Work out the finished part from the listing and answer in its coordinate system (mm). Face numbers are marked on the shaded views. A direction names the side the tool comes from. Coordinates: 2 decimals unless noted, no trailing zeros. Write each loop counter-clockwise with the first axis right and the second up, starting at its lowest first coordinate (ties: lowest second). Pieces come first, ordered by that corner, then holes. Notation, with made-up numbers: M 62.25,38 L 66.25,38 A17 ccw 66.25,51 Z; hole C 0.5,1 d8. An arc over 180 degrees is marked long. Use CSV: the item, a comma, the result in double quotes.
from build123d import *

# Parameters (mm, degrees)
F0_R     = 12.5
F1_DEPTH = 25
F2_R     = 5


with BuildPart() as f1:
    # F0 (on Front) → F1 (new body)
    with BuildSketch(Plane.XZ):
        with BuildLine():
            ThreePointArc((25.1206115917, 18.3788214192), (0, 57.0683197663), (-25.1206115917, 18.3788214192))
            Line((-25.1206115917, 18.3788214192), (-25.1206115917, -41.6211785808))
            Line((-25.1206115917, -41.6211785808), (25.1206115917, -41.6211785808))
            Line((25.1206115917, -41.6211785808), (25.1206115917, 18.3788214192))
        make_face()
        with Locations((0, 29.5683197663)):
            Circle(F0_R, mode=Mode.SUBTRACT)
    extrude(amount=F1_DEPTH)

    # F2
    f2_edges = [f1.edges().sort_by_distance(p)[0] for p in [
        (-25.120612, -12.5, -41.621179),
        (25.120612, -12.5, -41.621179),
        (-25.120612, -12.5, 18.378821),
        (25.120612, -12.5, 18.378821),
        (0, 0, 57.06832),
        (0, -25, 57.06832),
        (25.120612, 0, -11.621179),
        (25.120612, -25, -11.621179),
        (-25.120612, 0, -11.621179),
        (-25.120612, -25, -11.621179),
    ]]
    fillet(f2_edges, radius=F2_R)


solid = f1.part
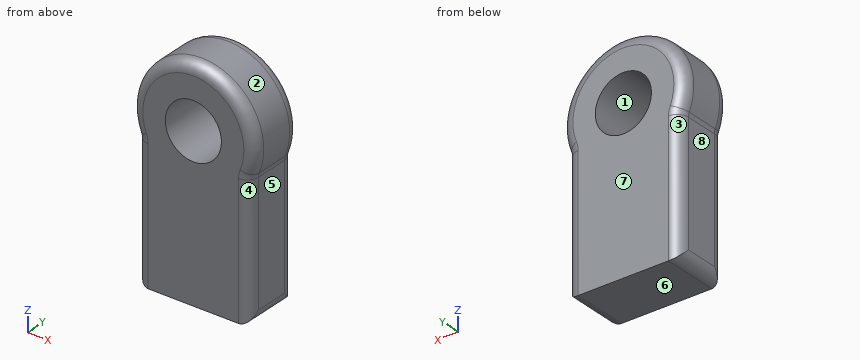
Item 1: Consider probe 1 along Z at (x, y) = (0, -8); probe 2 along X at (y, z) = (-8.25, 2.5); probe 3 along Z at (x, y) = (-10, -4.75). Determine where each line is inside the solid, lowest interval first.
Answer:
probe 1,"z = -41.62 to 17.07, 42.07 to 57.07"
probe 2,"x = -25.12 to 25.12"
probe 3,"z = -41.62 to 22.07, 37.07 to 55.18"
Item 2: A tool of negligible diameter and unlimited length cuts with its end or side. For the marked faces 4, 5, 6, 7 and 8, from which of +Z, -Z, +X, -X, +Y, -Y can it reach the whole face along a straight path? Write none if from no direction.
Answer:
face 4,"-Z, +X, -Y"
face 5,"-Z, +X, +Y, -Y"
face 6,"-Z, +X, -X, +Y, -Y"
face 7,"+Z, -Z, +X, -X, +Y"
face 8,"-Z, -X, +Y, -Y"
Item 3: The part is cut by section A-A (x = 0). Write down the section's boundary in (y, z).
Answer:
outline,"M -25,-41.62 L 0,-41.62 L 0,17.07 L -25,17.07 Z; M -25,42.07 L 0,42.07 L 0,52.07 A5 ccw -5,57.07 L -20,57.07 A5 ccw -25,52.07 Z"
Item 4: For a pull along X with two mould halves and no side action, classify the marked faces 1, 2 and 3 as released by +X, released by -X, zero draft, split by the parting line, or undercut.
Answer:
face 1,"undercut"
face 2,"split by the parting line"
face 3,"released by -X"
Item 5: The part is cut by section B-B (z = -34). Write down the section's boundary in (x, y), then the cut area to 3 significant figures.
Answer:
outline,"M -25.12,-20 A5 ccw -20.12,-25 L 20.12,-25 A5 ccw 25.12,-20 L 25.12,-5 A5 ccw 20.12,0 L -20.12,0 A5 ccw -25.12,-5 Z"
area,"1,230 mm2"
Item 6: Given pin 1 (4.5 mm diameter, centred on y = -12, z = 3.5, fed in from +X); pin 2 (10 mm diameter, centred on x = 10, y = -8.5, fed in from +Z); pin 3 (1.5 mm diameter, centred on y = -4.5, z = 44.5, fed in from +X), each flat-ended and moving along its own axis, determine where each tip first touches the part or whether it passes through.
Answer:
pin 1,"stops at x = 25.12"
pin 2,"stops at z = 56.61"
pin 3,"stops at x = 23.54"
Item 7: The part is cut by section C-C (y = -15.75). Write down the section's boundary in (x, z).
Answer:
outline,"M -25.49,19.24 A5 cw -25.12,17.36 L -25.12,-36.62 A5 ccw -20.12,-41.62 L 20.12,-41.62 A5 ccw 25.12,-36.62 L 25.12,17.36 A5 cw 25.49,19.24 A27.5 ccw long Z; hole C 0,29.57 d25"
Item 8: The part is cut by section D-D (y = -21). Write down the section's boundary in (x, z).
Answer:
outline,"M -25.39,19.28 A5.1 cw -25.02,17.36 L -25.02,-37.62 A5 ccw -20.12,-41.62 L 20.12,-41.62 A5 ccw 25.02,-37.62 L 25.02,17.36 A5.1 cw 25.39,19.28 A27.4 ccw long Z; hole C 0,29.57 d25"
